For this review, take the finished solid that the model builds, in its own axes (mm). Face numbers are marked on the shaded views. A direction names the side the tool comes from. Coordinates: 2 decimals unless noted, no trailing zeros. Order: outer loops, then holes, each group sorted by start corner. A loop starts at its lowest first (then second) coordinate and runs counter-clockwise, first axis right, second up. Notation, with made-up numbers: M 85.5,46.5 L 115.5,46.5 A23 ccw 115.5,78.5 Z; hole C 62.25,-16 d10. An arc over 180 degrees is marked long. Use one line per item in the form item = value. Start each with the question number.
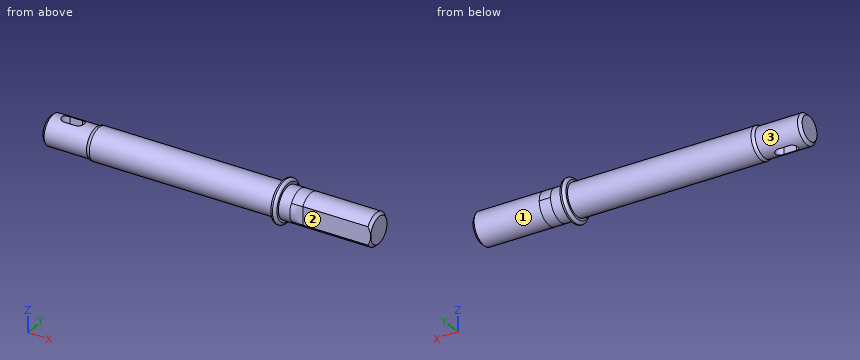
Autodesk Inventor part; units mm, degrees
ref_plane "Work Plane1" through (24, 0, 0) normal (1, 0, 0) x (0, 0, -1)
ref_plane "Work Plane2" through (19, 0, 0) normal (-1, 0, 0) x (0, 0, 1)
ref_plane "YZ Plane" through (0, 0, 0) normal (1, 0, 0) x (0, 1, 0)
sketch "Sketch1" plane through (0, 0, 0) normal (1, 0, 0) x (0, 1, 0)
  circle A0 centre (0, 0) radius 2.85
  dimension "diameter" = 5.7
extrude "Shaft" add sketch "Sketch1" along normal mid plane 44
sketch "Sketch2" plane through (0, 0, 0) normal (0, 0, 1) x (1, 0, 0)
  line L0 (-22, -2.85) -> (-22, 2.85) construction
  line L1 (22, -2.85) -> (-22, -2.85) construction
  line L2 (22, 2.85) -> (22, -2.85) construction
  line L3 (-22, 2.85) -> (22, 2.85) construction
  line L4 (-22, -2.85) -> (22, -2.85)
  line L5 (-15, -2.85) -> (-15, -2.85)
  line L6 (-22, -2.85) -> (22, -2.85)
  line L7 (-20, 0) -> (-16, 0) construction
  line L8 (-19.1, -0.9) -> (-16.9, -0.9)
  line L9 (-16.9, 0.9) -> (-19.1, 0.9)
  arc A0 (-19.1, 0.9) -> (-19.1, -0.9) centre (-19.1, 0) ccw
  arc A1 (-16.9, -0.9) -> (-16.9, 0.9) centre (-16.9, 0) ccw
  point P0 (0, 0)
  point P1 (22, 0)
  point P2 (-18, 0)
  dimension "d17" = 1.8
  dimension "d20" = 2
  dimension "d21" = 1
  dimension "d22" = 7
extrude "Slot for Differential Gear" cut sketch "Sketch2" along normal through all both and the other way through all
ref_plane "Work Plane1" through (24, 0, 0) normal (1, 0, 0) x (0, 0, -1)
sketch "Sketch3" plane through (24, 0, 0) normal (1, 0, 0) x (0, 0, -1)
  arc A0 (1.6583, -2.5) -> (-1.6583, -2.5) centre (0, 0) ccw construction
  circle A1 centre (0, 0) radius 2.85 construction
  line L0 (-1.6583, -2.5) -> (1.6583, -2.5)
  arc A2 (1.6125, -2.35) -> (-1.6125, -2.35) centre (0, 0) ccw
  line L1 (1.6125, -2.35) -> (-1.6125, -2.35)
  point P0 (-1.3684, -2.5)
  point P1 (1.3684, -2.5)
  dimension "d49" = 3
  dimension "d50" = 2.5
  dimension "wheel_offset" = 0.15
extrude "Wheel Insert Profile" add sketch "Sketch3" along normal blind 12
loft "Loft1" add section 1 edges at (22, -2.85, 0) section 2 edges at (24, -2.35, 0) (24, 2.85, 0)
ref_plane "Work Plane2" through (19, 0, 0) normal (-1, 0, 0) x (0, 0, 1)
sketch "Sketch4" plane through (19, 0, 0) normal (-1, 0, 0) x (0, 0, 1)
  circle A0 centre (0, 0) radius 3.75
  dimension "d35" = 7.5
extrude "Stopper" add sketch "Sketch4" against normal blind 1
fillet "Fillet1" radius 0.5 2 edges at (19, 0, -3.75) (20, 0, -3.75)
sketch "Sketch8" plane through (-22, 0, 0) normal (-1, 0, 0) x (0, 0, 1)
  circle A0 centre (0, 0) radius 2.85
  circle A1 centre (0, 0) radius 2.7 construction
  circle A2 centre (0, 0) radius 2.65
  dimension "d68" = 5.4
  dimension "d69" = 0.05
extrude "Differential Gear Insert Profile" cut sketch "Sketch8" against normal blind 8
fillet "Fillet3" radius 1 1 edges at (-14, -2.85, 0)
chamfer "Chamfer4" distance 0.5 angle 45 2 edges at (-22, 0, -2.65) (36, 2.85, 0)
properties part number "rear shaft v2"
1. Tool access review of the marked faces 1, 2 and 3: name each direction out of +Z, -Z, +X, -X, +Y, -Y from which nothing blocks a thin tool from reaching the whole face with its end or side.
2. For pin 1 Ø4 at (x, y) = (14, -2.5) entering from +Z; pin 2 Ø1.1 at (x, z) = (-18.5, 0.5) entering from +Y; pin 3 Ø1.1 at (x, z) = (-17.5, 0) entering from -Y, all flat-tipped, find the tip position at first contact; note any pin that passes through.
3. To check wall thickness, follow line 1 (X direction, y = -1, z = 3); line 2 (Y direction, x = 33.5, z = 0); line 3 (X direction, y = -0.5, z = -1.75). State the ranges of each line that lie inside material, in increasing order.
4. Consider section B-B, the plane x = 4. Write out the cut boundary in (y, z).
5. Consider section A-A, the plane x = 27.5. Write out the cut boundary in (y, z), plus the area to 3 significant figures.
Answers follow:
q1.face_1 = +X
q1.face_2 = +Z, -Z, +X, -Y
q1.face_3 = -X
q2.pin_1 = 2.81
q2.pin_2 = 2.65
q2.pin_3 = -2.65
q3.line_1 = 19 to 20
q3.line_2 = -2.35 to 2.85
q3.line_3 = -22 to -19.85, -16.15 to 36
q4.outline = C 0,0 d5.7
q5.outline = M -2.35,-1.61 A2.85 ccw long -2.35,1.61 Z
q5.area = 24.4 mm²
